from build123d import *

# Parameters (mm, degrees)
SKETCH1_R               = 2.5
BOSS_EXTRUDE1_DEPTH     = 4.3
SKETCH2_R               = 3
BOSS_EXTRUDE2_DEPTH     = 1
FILLET1_R               = 2.5
CUT_EXTRUDE1_DEPTH      = 7.040695324
CUT_EXTRUDE1_DEPTH_BACK = 7.040695324
SKETCH3_W               = 0.954190985
SKETCH3_H               = 1.425570426
SKETCH4_W               = 0.6
SKETCH4_H               = 0.6
BOSS_EXTRUDE3_DEPTH     = 27
SKETCH4_3_W             = 0.6
SKETCH4_3_H             = 0.6
BOSS_EXTRUDE4_DEPTH     = 25.5
FILLET2_R               = 0.15
FILLET3_R               = 0.15
FILLET4_R               = 0.15
FILLET5_R               = 0.15


with BuildPart() as part:
    # Sketch1 → Boss-Extrude1 (new, symmetric)
    with BuildSketch(Plane(origin=(0, 0, 0), x_dir=(1, 0, 0), z_dir=(0, 1, 0))):
        with Locations(Location((0, 0, 0), (0, 0, 90))):
            Circle(SKETCH1_R)
    extrude(amount=BOSS_EXTRUDE1_DEPTH, both=True)

    # Sketch2 → Boss-Extrude2 (add)
    with BuildSketch(Plane.XZ.offset(4.3)):
        with Locations(Location((0, 0, 0), (0, 0, 270))):
            Circle(SKETCH2_R)
    extrude(amount=-BOSS_EXTRUDE2_DEPTH)

    # Fillet1
    fillet1_edges = [part.edges().sort_by_distance(p)[0] for p in [
        (0, 4.3, 2.5),
    ]]
    fillet(fillet1_edges, radius=FILLET1_R)

    # Sketch3 → Cut-Extrude1 (cut, two sides: drawn at the far end of the back side and taken through both)
    with BuildSketch(Plane.XY.offset(-CUT_EXTRUDE1_DEPTH_BACK)):
        with Locations((2.977095493, -4.012785213)):
            Rectangle(SKETCH3_W, SKETCH3_H)
    extrude(amount=CUT_EXTRUDE1_DEPTH + CUT_EXTRUDE1_DEPTH_BACK, mode=Mode.SUBTRACT)

    # Sketch4 → Boss-Extrude3 (add)
    with BuildSketch(Plane.XZ.offset(4.3)):
        with Locations((-1.27, 0)):
            Rectangle(SKETCH4_W, SKETCH4_H)
    extrude(amount=BOSS_EXTRUDE3_DEPTH)

    # Sketch4_3 → Boss-Extrude4 (add)
    with BuildSketch(Plane.XZ.offset(4.3)):
        with Locations((1.27, 0)):
            Rectangle(SKETCH4_3_W, SKETCH4_3_H)
    extrude(amount=BOSS_EXTRUDE4_DEPTH)

    # Fillet2
    fillet2_edges = [part.edges().sort_by_distance(p)[0] for p in [
        (-0.97, -4.3, 0),
        (-1.27, -4.3, 0.3),
        (-1.27, -4.3, -0.3),
        (-1.57, -4.3, 0),
    ]]
    fillet(fillet2_edges, radius=FILLET2_R)

    # Fillet3
    fillet3_edges = [part.edges().sort_by_distance(p)[0] for p in [
        (0.97, -4.3, 0),
        (1.27, -4.3, -0.3),
        (1.27, -4.3, 0.3),
        (1.57, -4.3, 0),
    ]]
    fillet(fillet3_edges, radius=FILLET3_R)

    # Fillet4
    fillet4_edges = [part.edges().sort_by_distance(p)[0] for p in [
        (-1.27, -31.3, -0.3),
        (-1.57, -31.3, 0),
        (-0.97, -31.3, 0),
        (-1.27, -31.3, 0.3),
    ]]
    fillet(fillet4_edges, radius=FILLET4_R)

    # Fillet5
    fillet5_edges = [part.edges().sort_by_distance(p)[0] for p in [
        (1.57, -29.8, 0),
        (1.27, -29.8, 0.3),
        (0.97, -29.8, 0),
        (1.27, -29.8, -0.3),
    ]]
    fillet(fillet5_edges, radius=FILLET5_R)


solid = part.part
Design review of the part built by this model. Coordinates are the model's own, in mm. A direction names the side the tool comes from. Coordinates: 2 decimals unless noted, no trailing zeros. Loops run counter-clockwise (first coordinate to the right, second up) from the corner with the lowest first, then second, coordinate; pieces in that order, holes last. Notation, with made-up numbers: M 56,-2.5 L 62,-2.5 A17 ccw 62,9.5 Z; hole C 86,-12 d1. An arc over 180 degrees is marked long. Use one line per item in the form item = value.
(1) For line 1 along Y through (x, z) = (-0.45, -2.5); line 2 along X through (y, z) = (-3, 0.1); line 3 along Y through (x, z) = (1.6, 1.75), list the stretches that pass through material, from the lowest coordinate up. Write a range as from..to.
Return value:
line_1 = -4.3..-3.3
line_2 = -2.5..2.5
line_3 = -4.3..2.59
(2) For faces 1 (the face through (-3, -4, 0)), 2 (the face through (-2, -3.3, -2)), list the 3-axis set-ups (+Z, -Z, +X, -X, +Y, -Y) from which the entire face can be reached by the end or side of a thin tool; tool diameter is ignored.
Return value:
face_1 = +Y, -Y
face_2 = +Y
(3) Clearance check with flat-ended pins moving along their axes: P1, Ø0.5, axis at y = -22.5, z = 0, coming from the -X side; P2, Ø0.5, axis at x = 1.5, y = -23, coming from the -Z side; P3, Ø1.5, axis at y = -23, z = 0, coming from the +X side. State where each tip first meets the part, or that it passes through.
Return value:
P1 = -1.57
P2 = -0.3
P3 = 1.57
(4) Consider section C-C (y = -0.5). Write out the cut boundary in (x, z), and give its area (3 significant figures).
Return value:
outline = C 0,0 d5
area = 19.6 mm2
(5) Consider section B-B (x = 0). Write out the cut boundary in (y, z), and give its area (3 significant figures).
Return value:
outline = M -4.3,-3 L -3.3,-3 L -3.3,-2.5 L 1.8,-2.5 A2.5 ccw 1.8,2.5 L -3.3,2.5 L -3.3,3 L -4.3,3 Z
area = 41.3 mm2
(6) Consider section A-A (y = -8). Write out the cut boundary in (x, z), and give its area (3 significant figures).
Return value:
outline = M -1.57,-0.3 L -0.97,-0.3 L -0.97,0.3 L -1.57,0.3 Z; M 0.97,-0.3 L 1.57,-0.3 L 1.57,0.3 L 0.97,0.3 Z
area = 0.720 mm2
